```python
from build123d import *

# Parameters (mm, degrees)
BOSS_EXTRU_1_DEPTH      = 8
ESQUISSE2_R             = 40
ENL_V_MAT_EXTRU_1_DEPTH = 4
ESQUISSE4_R             = 10.5
BOSS_EXTRU_2_DEPTH      = 40
ESQUISSE5_R             = 8.5
ENL_V_MAT_EXTRU_2_DEPTH = 40
CONG_1_R                = 5
CONG_4_R                = 2


with BuildPart() as part:
    # Esquisse1 → Boss.-Extru.1 (new body)
    with BuildSketch(Plane(origin=(0, 0, 0), x_dir=(1, 0, 0), z_dir=(0, 1, 0))):
        with BuildLine():
            Line((-30, -33.541019662), (-46.666666667, -52.174919475))
            ThreePointArc((-46.666666667, -52.174919475), (0, -70), (46.666666667, -52.174919475))
            Line((46.666666667, -52.174919475), (30, -33.541019662))
            ThreePointArc((30, -33.541019662), (0, 45), (-30, -33.541019662))
        make_face()
    extrude(amount=BOSS_EXTRU_1_DEPTH)

    # Esquisse2 → Enlèv. mat.-Extru.1 (cut)
    with BuildSketch(Plane(origin=(0, 8, 0), x_dir=(1, 0, 0), z_dir=(0, 1, 0))):
        with Locations(Location((0, 0, 0), (0, 0, 270))):
            Circle(ESQUISSE2_R)
    extrude(amount=-ENL_V_MAT_EXTRU_1_DEPTH, mode=Mode.SUBTRACT)

    # Esquisse4 → Boss.-Extru.2 (add)
    with BuildSketch(Plane(origin=(0, 8, 0), x_dir=(1, 0, 0), z_dir=(0, 1, 0))):
        with Locations(Location((0, -55, 0), (0, 0, 270))):
            Circle(ESQUISSE4_R)
        with Locations(Location((-24.5, -49.241750578, 0), (0, 0, 270))):
            Circle(ESQUISSE4_R)
        with Locations(Location((24.5, -49.241750578, 0), (0, 0, 90))):
            Circle(ESQUISSE4_R)
    extrude(amount=BOSS_EXTRU_2_DEPTH)

    # Esquisse5 → Enlèv. mat.-Extru.2 (cut)
    with BuildSketch(Plane(origin=(0, 48, 0), x_dir=(1, 0, 0), z_dir=(0, 1, 0))):
        with Locations(Location((0, -55, 0), (0, 0, 270))):
            Circle(ESQUISSE5_R)
        with Locations(Location((-24.5, -49.241750578, 0), (0, 0, 270))):
            Circle(ESQUISSE5_R)
        with Locations(Location((24.5, -49.241750578, 0), (0, 0, 270))):
            Circle(ESQUISSE5_R)
    extrude(amount=-ENL_V_MAT_EXTRU_2_DEPTH, mode=Mode.SUBTRACT)

    # Congé1
    cong_1_edges = [part.edges().sort_by_distance(p)[0] for p in [
        (30, 4, 33.541019662),
        (46.666666667, 4, 52.174919475),
        (-46.666666667, 4, 52.174919475),
        (-30, 4, 33.541019662),
    ]]
    fillet(cong_1_edges, radius=CONG_1_R)

    # Congé4
    cong_4_edges = [part.edges().sort_by_distance(p)[0] for p in [
        (0, 8, 44.5),
        (-24.5, 8, 38.741750578),
        (24.5, 8, 59.741750578),
    ]]
    fillet(cong_4_edges, radius=CONG_4_R)


solid = part.part
```
Here's how the part is built. I have some questions about the finished solid (model axes, mm). A direction names the side the tool comes from. Round coordinates to 2 decimals unless told otherwise and drop trailing zeros. Write each loop counter-clockwise with the first axis right and the second up, starting at its lowest first coordinate (ties: lowest second). Pieces come first, ordered by that corner, then holes.
Q1. If we section it at A-A on y = 23.5: Write out the boundary of the cut face in (x, z), plus the area to 3 significant figures.
Q2. Which directions (+Z, -Z, +X, -X, +Y, -Y) give clear straight access to the entire face, cutting with the end or side of a thin tool? Please do faces 1 (the flat face through (-38.1, 3.9, 42.6)), 2 (the cylindrical face through (-39.05, 6.03, -8.67)), 3 (the flat face through (38.256, 3.944, 42.771)).
Q3. If we section it at B-B on x = 0: Write out the boundary of the cut face in (y, z).
Q4. If we section it at C-C on z = 25: Write out the boundary of the cut face in (x, y).
Q5. If we mould it in two halves opening along X, with no side actions, what happens to faces 4 (the flat face through (-1, 0, 12)), 5 (the cylindrical face through (31.894, 4.056, 33.668)), 6 (the cylindrical face through (-17.404, 28.734, 41.503)), 7 (the cylindrical face through (0.46, 28.73, 44.51))? For each: +X half, -X half, draft (parallel to the pull), parting line (faces both ways), or undercut.
Q6. If we section it at D-D on x = -24.5: Write out the boundary of the cut face in (y, z), plus the area to 3 significant figures.
Q7. Will these pins go through, and if not, where does the flat tip stop? P1, Ø10, axis at x = 9, y = 6, coming from the +Z side; P2, Ø4, axis at y = 6.5, z = 34.5, coming from the -X side; P3, Ø12, axis at x = 31.5, y = 24.5, coming from the +Z side.
Q8. Please list where these lines run through material, in increasing order: probe 1 along X at (y, z) = (7, -1); probe 2 along X at (y, z) = (43, 53.5); probe 3 along Y at (x, z) = (15.5, -16).
Answer below:
1. outline: circle Ø21 at (-24.5, 49.24); circle Ø21 at (0, 55); circle Ø21 at (24.5, 49.24); hole circle Ø17 at (-24.5, 49.24); hole circle Ø17 at (0, 55); hole circle Ø17 at (24.5, 49.24)
1. area: 358 mm2
2. face 1: -X, +Y, -Y
2. face 2: +Y
2. face 3: +X, +Y, -Y
3. outline: (0, -45) - (8, -45) - (8, -40) - (4, -40) - (4, 40) - (8, 40) - (8, 42.5) arc R2 cw to (10, 44.5) - (48, 44.5) - (48, 46.5) - (8, 46.5) - (8, 63.5) - (48, 63.5) - (48, 65.5) - (10, 65.5) arc R2 cw to (8, 67.5) - (8, 70) - (0, 70) - close
4. outline: (-37.42, 0) - (37.42, 0) - (37.42, 8) - (31.22, 8) - (31.22, 4) - (-31.22, 4) - (-31.22, 8) - (-37.42, 8) - close
5. face 4: draft
5. face 5: +X half
5. face 6: undercut
5. face 7: undercut
6. outline: (0, -37.75) - (8, -37.75) - (8, -31.62) - (4, -31.62) - (4, 31.62) - (8, 31.62) - (8, 36.74) arc R2 cw to (10, 38.74) - (48, 38.74) - (48, 40.74) - (8, 40.74) - (8, 57.74) - (48, 57.74) - (48, 59.74) - (10, 59.74) arc R2 cw to (8, 61.74) - (8, 65.57) - (0, 65.57) - close
6. area: 735 mm2
7. P1: stops at z = 69.89
7. P2: stops at x = -32.72
7. P3: stops at z = 59.69
8. probe 1: x = -44.99 to -39.99, 39.99 to 44.99
8. probe 2: x = -34.1 to -31.86, -17.14 to -14.9, -10.39 to -8.37, 8.37 to 10.39, 14.9 to 17.14, 31.86 to 34.1
8. probe 3: y = 0 to 4
